```python
from build123d import *

# Parameters (mm, degrees)
EXTRUDE_1_DEPTH     = 12
CHAMFER_1_SIZE      = 0.2
SKETCH_2_R          = 1.5
CUT_EXTRUDE_1_DEPTH = 28.057584889
CHAMFER_2_SIZE      = 1


with BuildPart() as part:
    # 草图1 → 凸台-拉伸1 (new body)
    with BuildSketch(Plane.XY):
        Polygon((0, 0), (0, 22.27), (9.6, 22.27), (9.6, 17.27), (8.3, 17.27), (8.3, 15.77), (3, 15.77), (3, 5), (9.6, 5), (9.6, 0), align=None)
    extrude(amount=EXTRUDE_1_DEPTH)

    # 倒角1
    chamfer_1_edges = [part.edges().sort_by_distance(p)[0] for p in [
        (8.3, 15.77, 6),
    ]]
    chamfer(chamfer_1_edges, length=CHAMFER_1_SIZE)

    # 草图2 → 切除-拉伸1 (cut, through all)
    with BuildSketch(Plane.ZY):
        with Locations((9.5, 19.77)):
            Circle(SKETCH_2_R)
        with Locations((2.5, 19.77)):
            Circle(SKETCH_2_R)
        with Locations((2.5, 2.5)):
            Circle(SKETCH_2_R)
        with Locations((9.5, 2.5)):
            Circle(SKETCH_2_R)
    extrude(amount=-CUT_EXTRUDE_1_DEPTH, mode=Mode.SUBTRACT)

    # 倒角2
    chamfer_2_edges = [part.edges().sort_by_distance(p)[0] for p in [
        (0, 0, 6),
        (0, 22.27, 6),
    ]]
    chamfer(chamfer_2_edges, length=CHAMFER_2_SIZE - 0.0001)  # a hair under: the kernel refuses the full size


solid = part.part
```
Input: part model. Units: mm. Frame: model coordinates. A direction names the side the tool comes from. Give positions to 0.01 mm unless a question says otherwise; leave off trailing zeros. Order: outer loops, then holes, each group sorted by start corner. A loop starts at its lowest first (then second) coordinate and runs counter-clockwise, first axis right, second up. Notation, with made-up numbers: (-38, 11) - (-34, 11) arc R27 cw to (-34, 35) - close; hole circle Ø8 at (69, 56.5). An arc over 180 degrees is marked (long way). One line per item, written item: value.
1. Cut plane D-D, the plane x = 1.25. Output: boundary loops of the cut face in (y, z), and give its area (3 significant figures).
Determined:
outline: (0, 0) - (22.27, 0) - (22.27, 12) - (0, 12) - close; hole circle Ø3 at (2.5, 2.5); hole circle Ø3 at (2.5, 9.5); hole circle Ø3 at (19.77, 2.5); hole circle Ø3 at (19.77, 9.5)
area: 239 mm2
2. Cut plane B-B, the plane z = 9.5. Give the number of separate pieces and of enclosed holes in the cut face, and give its area (3 significant figures).
Determined:
separate pieces: 3
enclosed holes: 0
area: 82.1 mm2
3. Line query: probe 1 along Y at (x, z) = (7, 9.5); probe 2 along Y at (x, z) = (2.75, 2.5); probe 3 along Y at (x, z) = (0.75, 2.5). Output: solid intervals per line, ascending.
Determined:
probe 1: 0 to 1, 4 to 5, 15.77 to 18.27, 21.27 to 22.27
probe 2: 0 to 1, 4 to 18.27, 21.27 to 22.27
probe 3: 0.25 to 1, 4 to 18.27, 21.27 to 22.02
4. Pin query (flat end, axial travel): pin 1 Ø1 at (y, z) = (7, 2) entering from +X; pin 2 Ø1.5 at (x, y) = (8.5, 14) entering from -Z. Return the tip coordinate at first contact, or that it passes through.
Determined:
pin 1: x = 3
pin 2: through
5. Cut plane A-A, the plane x = 9. Output: boundary loops of the cut face in (y, z), and give its area (3 significant figures).
Determined:
outline: (0, 0) - (5, 0) - (5, 12) - (0, 12) - close; (17.27, 0) - (22.27, 0) - (22.27, 12) - (17.27, 12) - close; hole circle Ø3 at (2.5, 2.5); hole circle Ø3 at (2.5, 9.5); hole circle Ø3 at (19.77, 2.5); hole circle Ø3 at (19.77, 9.5)
area: 91.7 mm2
6. Cut plane C-C, the plane y = 2.5. Output: boundary loops of the cut face in (x, z), and give its area (3 significant figures).
Determined:
outline: (0, 0) - (9.6, 0) - (9.6, 1) - (0, 1) - close; (0, 4) - (9.6, 4) - (9.6, 8) - (0, 8) - close; (0, 11) - (9.6, 11) - (9.6, 12) - (0, 12) - close
area: 57.6 mm2
7. Draft query along Z for faces 3 (the face through (4.733, 1.036, 2.175)), 4 (the face through (0, 11, 6)), 5 (the face through (2.7, 11.3, 0)). Return one class per face: released by +Z, released by -Z, zero draft, split by the parting line, or undercut.
Determined:
face 3: undercut
face 4: zero draft
face 5: released by -Z
8. Reachability of faces 1 (the face through (9, 17.27, 6)), 2 (the face through (9.6, 20, 6)) from +Z, -Z, +X, -X, +Y, -Y: full face, straight path, thin tool, end or side. Return the list, or none.
Determined:
face 1: +Z, -Z, +X
face 2: +Z, -Z, +X, +Y, -Y
